Part model, mm, in its own coordinate system. Round coordinates to 2 decimals unless told otherwise and drop trailing zeros. Loops run counter-clockwise (first coordinate to the right, second up) from the corner with the lowest first, then second, coordinate; pieces in that order, holes last. Notation, with made-up numbers: M 3,-7 L 50,-7 A38 cw 50,32 Z; hole C 9.5,70.5 d4. An arc over 180 degrees is marked long. Put each result on its own line as item: value. Start each with the question number.
1) Slice it at A-A on x = 88.9. Give the cut face in (y, z), then the cut area to 3 significant figures.
2) Probe line 1 along Y through (x, z) = (88.9, 1.1); line 2 along X through (y, z) = (22.5, 0.1); line 3 along Y through (x, z) = (65, 1.6). List the from-to ranges inside material, lowest first.
3) Slice it at B-B on y = 57.15. Give the cut face in (x, z).
4) Slice it at D-D on x = 154.5. Give the cut face in (y, z).
5) Drop a flat-ended pin along its axis: pin 1 Ø1 at (y, z) = (108.5, 2) entering from +X. Give the stop position or say it passes through.
6) Slice it at C-C on y = 112.5. Give the cut face in (x, z), then the cut area to 3 significant figures.
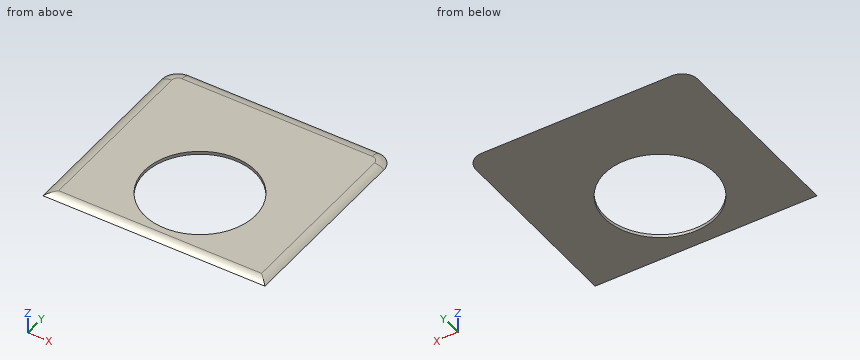
```python
from build123d import *

# Parameters (mm, degrees)
SKETCH1_W           = 177.8
SKETCH1_H           = 160.528
SKETCH1_R           = 44.45
BOSS_EXTRUDE1_DEPTH = 2.54
FILLET1_R           = 12.7
FILLET2_R           = 12.7


with BuildPart() as part:
    # Sketch1 → Boss-Extrude1 (new body)
    with BuildSketch(Plane.XY):
        with Locations((88.9, 80.264)):
            Rectangle(SKETCH1_W, SKETCH1_H)
        with Locations((88.9, 57.15)):
            Circle(SKETCH1_R, mode=Mode.SUBTRACT)
    extrude(amount=BOSS_EXTRUDE1_DEPTH)

    # Fillet1
    fillet1_edges = [part.edges().sort_by_distance(p)[0] for p in [
        (0, 160.528, 1.27),
        (177.8, 160.528, 1.27),
    ]]
    fillet(fillet1_edges, radius=FILLET1_R)

    # Fillet2
    # the kernel refuses this fillet: 12.7 mm, written as the material it takes off along each edge
    with BuildSketch(Plane(origin=(177.8, -19.05, 2.54), x_dir=(0, 0, -1), z_dir=(0, 1, 0))) as fillet2_piece_1:
        with BuildLine():
            CenterArc((12.7, 7.62), FILLET2_R, 180, 36.869897646)
            Line((0, 7.62), (-0.254, 7.62))
            Line((-0.254, 7.62), (-0.254, 0))
            Line((-0.254, 0), (0, -0.254))
            ThreePointArc((0, -0.254), (1.27, -0.254), (2.3368, -0.1524))
            Line((2.3368, -0.1524), (2.54, 0))
        make_face()
    extrude(amount=166.878, mode=Mode.SUBTRACT)
    with BuildSketch(Plane(origin=(165.1, 147.828, 2.54), x_dir=(1, 0, 0), z_dir=(0, -1, 0))) as fillet2_piece_2:
        with BuildLine():
            CenterArc((5.08, -12.7), FILLET2_R, 53.130102354, 36.869897646)
            Line((5.08, 0), (5.08, 0.254))
            Line((5.08, 0.254), (12.7, 0.254))
            Line((12.7, 0.254), (12.954, 0))
            ThreePointArc((12.954, 0), (12.954, -1.27), (12.8524, -2.3368))
            Line((12.8524, -2.3368), (12.7, -2.54))
        make_face()
    revolve(axis=Axis((165.1, 147.828, 2.54), (0, 0, 1)), revolution_arc=90, mode=Mode.SUBTRACT)
    with BuildSketch(Plane(origin=(165.1, 160.528, 2.54), x_dir=(0, -1, 0), z_dir=(-1, 0, 0))) as fillet2_piece_3:
        with BuildLine():
            CenterArc((7.62, -12.7), FILLET2_R, 90, 36.869897646)
            Line((0, -2.54), (-0.1524, -2.3368))
            ThreePointArc((-0.1524, -2.3368), (-0.254, -1.27), (-0.254, 0))
            Line((-0.254, 0), (0, 0.254))
            Line((0, 0.254), (7.62, 0.254))
            Line((7.62, 0.254), (7.62, 0))
        make_face()
    extrude(amount=152.4, mode=Mode.SUBTRACT)
    with BuildSketch(Plane(origin=(12.7, 147.828, 2.54), x_dir=(0, 1, 0), z_dir=(1, 0, 0))) as fillet2_piece_4:
        with BuildLine():
            CenterArc((5.08, -12.7), FILLET2_R, 53.130102354, 36.869897646)
            Line((12.7, -2.54), (12.8524, -2.3368))
            ThreePointArc((12.8524, -2.3368), (12.954, -1.27), (12.954, 0))
            Line((12.954, 0), (12.7, 0.254))
            Line((12.7, 0.254), (5.08, 0.254))
            Line((5.08, 0.254), (5.08, 0))
        make_face()
    revolve(axis=Axis((12.7, 147.828, 2.54), (0, 0, 1)), revolution_arc=90, mode=Mode.SUBTRACT)
    with BuildSketch(Plane(origin=(0, 147.828, 2.54), x_dir=(1, 0, 0), z_dir=(0, -1, 0))) as fillet2_piece_5:
        with BuildLine():
            CenterArc((7.62, -12.7), FILLET2_R, 90, 36.869897646)
            Line((0, -2.54), (-0.1524, -2.3368))
            ThreePointArc((-0.1524, -2.3368), (-0.254, -1.27), (-0.254, 0))
            Line((-0.254, 0), (0, 0.254))
            Line((0, 0.254), (7.62, 0.254))
            Line((7.62, 0.254), (7.62, 0))
        make_face()
    extrude(amount=166.878, mode=Mode.SUBTRACT)
    with BuildSketch(Plane(origin=(-19.05, 0, 2.54), x_dir=(0, 0, -1), z_dir=(1, 0, 0))) as fillet2_piece_6:
        with BuildLine():
            CenterArc((12.7, 7.62), FILLET2_R, 180, 36.869897646)
            Line((0, 7.62), (-0.254, 7.62))
            Line((-0.254, 7.62), (-0.254, 0))
            Line((-0.254, 0), (0, -0.254))
            ThreePointArc((0, -0.254), (1.27, -0.254), (2.3368, -0.1524))
            Line((2.3368, -0.1524), (2.54, 0))
        make_face()
    extrude(amount=215.9, mode=Mode.SUBTRACT)


solid = part.part
```
Recorded:
1. outline: M 0,0 L 12.7,0 L 12.7,2.54 L 7.62,2.54 A12.7 ccw Z; M 101.6,0 L 160.53,0 A12.7 ccw 152.91,2.54 L 101.6,2.54 Z
1. area: 170 mm2
2. line 1: y = 1.75 to 12.7, 101.6 to 158.78
2. line 2: x = 0.14 to 61.06, 116.74 to 177.66
2. line 3: y = 2.82 to 19.67, 94.63 to 157.7
3. outline: M 0,0 L 44.45,0 L 44.45,2.54 L 7.62,2.54 A12.7 ccw Z; M 133.35,0 L 177.8,0 A12.7 ccw 170.18,2.54 L 133.35,2.54 Z
4. outline: M 0,0 L 160.53,0 A12.7 ccw 152.91,2.54 L 7.62,2.54 A12.7 ccw Z
5. pin 1: stops at x = 175.21
6. outline: M 0,0 L 177.8,0 A12.7 ccw 170.18,2.54 L 7.62,2.54 A12.7 ccw Z
6. area: 439 mm2
